Part model, mm, in its own coordinate system. Face numbers are marked on the shaded views. A direction names the side the tool comes from. Round coordinates to 2 decimals unless told otherwise and drop trailing zeros. Write each loop counter-clockwise with the first axis right and the second up, starting at its lowest first coordinate (ties: lowest second). Pieces come first, ordered by that corner, then holes. Notation, with made-up numbers: (-27, 77.25) -> (4, 77.25) arc R36 ccw to (4, 116.25) -> close; hole circle Ø7 at (-31.5, 12). An arc over 180 degrees is marked (long way). Return JSON: item names as keys, results as strings. Group by question number.
(1) Tool access for the marked faces 5, 6 and 7: list every direction of +Z, -Z, +X, -X, +Y, -Y with a clear straight run to the whole face (end or side of a thin tool).
(2) Saw through at A-A (y = 0). List the corners of the cut face in (x, z) (3 decimals), plus the area to 3 significant figures.
(3) Saw through at C-C (z = 1.9). State how many separate pieces and enclosed holes the cut face has, plus the area to 3 significant figures.
(4) Drill centre lines: L1, parallel to Y at x = 14.85, z = 2.25 (3 decimals); L2, parallel to X at y = 7.25, z = 1.5 (3 decimals); L3, parallel to Y at x = -6, z = 0.3 (3 decimals). Where is each one in solid material? Low to high. Write a range as from..to.
(5) Mould opens along Y. For the marked faces 1, 2, 3 and 4 say: +Y half, -Y half, draft (parallel to the pull), parting line (faces both ways), or undercut.
(6) Saw through at B-B (x = 0). List the corners of the cut face in (y, z) (3 decimals).
(7) Drop flat-ended pins along their axis: pin 1 Ø2.5 at (x, y) = (-14.375, 11.375) entering from -Z; pin 2 Ø2.5 at (y, z) = (5.49, 2.25) entering from +X (3 decimals); pin 3 Ø1 at (x, y) = (0.5, -6.5) entering from +Z; pin 4 Ø1.6 at (x, z) = (0, 4) entering from -Y. Give the stop position or say it passes through.
Autodesk Inventor part; units mm, degrees
ref_plane "YZ Plane" through (0, 0, 0) normal (1, 0, 0) x (0, 1, 0)
ref_plane "XZ Plane" through (0, 0, 0) normal (0, 1, 0) x (-1, 0, 0)
ref_plane "XY Plane" through (0, 0, 0) normal (0, 0, 1) x (1, 0, 0)
ref_plane "Work Plane1" through (0, 0, 0) normal (0, 0, 1) x (1, 0, 0)
sketch "Sketch1" plane through (0, 0, 0) normal (0, 0, 1) x (1, 0, 0)
  arc A0 (5.9062, 3.651) -> (7.7035, 4.7619) centre (6.8048, 4.2064) ccw
  arc A1 (5.9062, 3.651) -> (2.5768, 6.4477) centre (0, 0) ccw
  arc A2 (3.3608, 8.4097) -> (2.5768, 6.4477) centre (2.9688, 7.4287) ccw
  arc A3 (7.7035, 4.7619) -> (3.3608, 8.4097) centre (0, 0) ccw
  arc A4 (2.5768, -6.4477) -> (3.3608, -8.4097) centre (2.9688, -7.4287) ccw
  arc A5 (2.5768, -6.4477) -> (5.9062, -3.651) centre (0, 0) ccw
  arc A6 (7.7035, -4.7619) -> (5.9062, -3.651) centre (6.8048, -4.2064) ccw
  arc A7 (3.3608, -8.4097) -> (7.7035, -4.7619) centre (0, 0) ccw
  arc A8 (-2.5553, 6.4563) -> (-3.3328, 8.4209) centre (-2.9441, 7.4386) ccw
  arc A9 (-2.5553, 6.4563) -> (-5.9062, 3.651) centre (0, 0) ccw
  arc A10 (-7.7035, 4.7619) -> (-5.9062, 3.651) centre (-6.8048, 4.2064) ccw
  arc A11 (-3.3328, 8.4209) -> (-7.7035, 4.7619) centre (0, 0) ccw
  arc A12 (-5.9062, -3.651) -> (-7.7035, -4.7619) centre (-6.8048, -4.2064) ccw
  arc A13 (-5.9062, -3.651) -> (-2.5553, -6.4563) centre (0, 0) ccw
  arc A14 (-3.3328, -8.4209) -> (-2.5553, -6.4563) centre (-2.9441, -7.4386) ccw
  arc A15 (-7.7035, -4.7619) -> (-3.3328, -8.4209) centre (0, 0) ccw
  circle A16 centre (0.0124, -10.65) radius 1.15
  circle A17 centre (8, 0) radius 1.0564
  circle A18 centre (-8, 0) radius 1.0564
  circle A19 centre (0, 0) radius 5
  circle A20 centre (0, 0) radius 13.7
  line L0 (16.125, 14.375) -> (-17.375, 14.375)
  line L1 (-17.375, 14.375) -> (-17.375, -14.375)
  line L2 (-17.375, -14.375) -> (16.125, -14.375)
  line L3 (16.125, -14.375) -> (16.125, 14.375)
  circle A21 centre (0, 0) radius 13.7
  circle A22 centre (0, 0) radius 5.15
  arc A23 (5.4809, 3.3881) -> (8.1288, 5.0248) centre (6.8048, 4.2064) ccw
  arc A24 (5.4809, 3.3881) -> (2.3912, 5.9835) centre (0, 0) ccw
  arc A25 (3.5464, 8.874) -> (2.3912, 5.9835) centre (2.9688, 7.4287) ccw
  arc A26 (8.1288, 5.0248) -> (3.5464, 8.874) centre (0, 0) ccw
  arc A27 (8.1288, -5.0248) -> (5.4809, -3.3881) centre (6.8048, -4.2064) ccw
  arc A28 (2.3912, -5.9835) -> (5.4809, -3.3881) centre (0, 0) ccw
  arc A29 (2.3912, -5.9835) -> (3.5464, -8.874) centre (2.9688, -7.4287) ccw
  arc A30 (3.5464, -8.874) -> (8.1288, -5.0248) centre (0, 0) ccw
  circle A31 centre (0.0124, -10.65) radius 1.65
  arc A32 (-5.4809, -3.3881) -> (-2.3713, -5.9914) centre (0, 0) ccw
  arc A33 (-5.4809, -3.3881) -> (-8.1288, -5.0248) centre (-6.8048, -4.2064) ccw
  arc A34 (-8.1288, -5.0248) -> (-3.5168, -8.8858) centre (0, 0) ccw
  arc A35 (-3.5168, -8.8858) -> (-2.3713, -5.9914) centre (-2.9441, -7.4386) ccw
  arc A36 (-2.3713, 5.9914) -> (-5.4809, 3.3881) centre (0, 0) ccw
  arc A37 (-2.3713, 5.9914) -> (-3.5168, 8.8858) centre (-2.9441, 7.4386) ccw
  arc A38 (-3.5168, 8.8858) -> (-8.1288, 5.0248) centre (0, 0) ccw
  arc A39 (-8.1288, 5.0248) -> (-5.4809, 3.3881) centre (-6.8048, 4.2064) ccw
  circle A40 centre (-14.375, -11.375) radius 1.75
  circle A41 centre (13.125, 11.375) radius 1.75
  circle A42 centre (13.125, -11.375) radius 1.75
  circle A43 centre (-14.375, 11.375) radius 1.75
  point P0 (0, 0)
  dimension "d0" = 0.15
  dimension "d1" = 0.5
  dimension "d2" = 0.5
  dimension "d3" = 0.5
  dimension "d4" = 0.5
  dimension "d5" = 0.5
extrude "Extrusion1" add sketch "Sketch1" along normal blind 1.5 contours A20 | L3 L2 L1 L0 | A40 | A41 | A42 | A43
sketch "Sketch2" plane through (0, 0, 1.5) normal (0, 0, 1) x (1, 0, 0)
  line L0 (-17.375, 14.375) -> (-17.375, -14.375)
  line L1 (-17.375, -14.375) -> (16.125, -14.375)
  line L2 (16.125, -14.375) -> (16.125, 14.375)
  line L3 (16.125, 14.375) -> (-17.375, 14.375)
  circle A0 centre (8, 0) radius 1.0564
  circle A1 centre (-8, 0) radius 1.0564
  circle A2 centre (0, 0) radius 5.15
  arc A3 (5.4809, 3.3881) -> (2.3912, 5.9835) centre (0, 0) ccw
  arc A4 (3.5464, 8.874) -> (2.3912, 5.9835) centre (2.9688, 7.4287) ccw
  arc A5 (8.1288, 5.0248) -> (3.5464, 8.874) centre (0, 0) ccw
  arc A6 (5.4809, 3.3881) -> (8.1288, 5.0248) centre (6.8048, 4.2064) ccw
  arc A7 (2.3912, -5.9835) -> (5.4809, -3.3881) centre (0, 0) ccw
  arc A8 (8.1288, -5.0248) -> (5.4809, -3.3881) centre (6.8048, -4.2064) ccw
  arc A9 (3.5464, -8.874) -> (8.1288, -5.0248) centre (0, 0) ccw
  arc A10 (2.3912, -5.9835) -> (3.5464, -8.874) centre (2.9688, -7.4287) ccw
  circle A11 centre (0.0124, -10.65) radius 1.65
  arc A12 (-5.4809, -3.3881) -> (-8.1288, -5.0248) centre (-6.8048, -4.2064) ccw
  arc A13 (-5.4809, -3.3881) -> (-2.3713, -5.9914) centre (0, 0) ccw
  arc A14 (-3.5168, -8.8858) -> (-2.3713, -5.9914) centre (-2.9441, -7.4386) ccw
  arc A15 (-8.1288, -5.0248) -> (-3.5168, -8.8858) centre (0, 0) ccw
  arc A16 (-2.3713, 5.9914) -> (-3.5168, 8.8858) centre (-2.9441, 7.4386) ccw
  arc A17 (-2.3713, 5.9914) -> (-5.4809, 3.3881) centre (0, 0) ccw
  arc A18 (-8.1288, 5.0248) -> (-5.4809, 3.3881) centre (-6.8048, 4.2064) ccw
  arc A19 (-3.5168, 8.8858) -> (-8.1288, 5.0248) centre (0, 0) ccw
  arc A20 (8.1288, -5.0248) -> (5.4809, -3.3881) centre (6.8048, -4.2064) ccw
  line L4 (8.3613, -4.2064) -> (8.3613, -14.375)
  line L5 (-17.375, -14.375) -> (16.125, -14.375)
  arc A21 (-5.4809, -3.3881) -> (-8.1288, -5.0248) centre (-6.8048, -4.2064) ccw
  line L6 (-8.3613, -4.2064) -> (-8.3613, -14.375)
  arc A22 (2.3912, -5.9835) -> (3.5464, -8.874) centre (2.9688, -7.4287) ccw
  line L7 (1.6624, -6.5827) -> (-1.6441, -6.5827)
  arc A23 (-3.5168, -8.8858) -> (-2.3713, -5.9914) centre (-2.9441, -7.4386) ccw
  point P0 (0, 0)
extrude "Extrusion2" add sketch "Sketch2" along normal blind 1.5 contours L3 L2 L1 L4 A8 A7 A10 L7 A14 A13 A12 L6 L0
sketch "Sketch3" plane through (0, 0, 3) normal (0, 0, 1) x (1, 0, 0)
  circle A0 centre (0, 0) radius 6.75
  line L0 (-17.375, -14.375) -> (-8.3613, -14.375)
  line L1 (-8.3613, -14.375) -> (-8.3613, -4.2064)
  arc A1 (-5.4809, -3.3881) -> (-8.3613, -4.2064) centre (-6.8048, -4.2064) ccw
  arc A2 (-5.4809, -3.3881) -> (-2.3713, -5.9914) centre (0, 0) ccw
  arc A3 (-1.6441, -6.5827) -> (-2.3713, -5.9914) centre (-2.9441, -7.4386) ccw
  line L2 (-1.6441, -6.5827) -> (1.6624, -6.5827)
  arc A4 (2.3912, -5.9835) -> (1.6624, -6.5827) centre (2.9688, -7.4287) ccw
  arc A5 (2.3912, -5.9835) -> (5.4809, -3.3881) centre (0, 0) ccw
  arc A6 (8.3613, -4.2064) -> (5.4809, -3.3881) centre (6.8048, -4.2064) ccw
  line L3 (8.3613, -4.2064) -> (8.3613, -14.375)
  line L4 (8.3613, -14.375) -> (16.125, -14.375)
  line L5 (16.125, -14.375) -> (16.125, 14.375)
  line L6 (16.125, 14.375) -> (-17.375, 14.375)
  line L7 (-17.375, 14.375) -> (-17.375, -14.375)
  circle A7 centre (8, 0) radius 1.0564
  circle A8 centre (-8, 0) radius 1.0564
  arc A9 (-2.3713, 5.9914) -> (-5.4809, 3.3881) centre (0, 0) ccw
  arc A10 (-8.1288, 5.0248) -> (-5.4809, 3.3881) centre (-6.8048, 4.2064) ccw
  arc A11 (-3.5168, 8.8858) -> (-8.1288, 5.0248) centre (0, 0) ccw
  arc A12 (-2.3713, 5.9914) -> (-3.5168, 8.8858) centre (-2.9441, 7.4386) ccw
  arc A13 (5.4809, 3.3881) -> (8.1288, 5.0248) centre (6.8048, 4.2064) ccw
  arc A14 (5.4809, 3.3881) -> (2.3912, 5.9835) centre (0, 0) ccw
  arc A15 (3.5464, 8.874) -> (2.3912, 5.9835) centre (2.9688, 7.4287) ccw
  arc A16 (8.1288, 5.0248) -> (3.5464, 8.874) centre (0, 0) ccw
  circle A17 centre (0, 0) radius 5.15
  circle A18 centre (8, 0) radius 2.5
  circle A19 centre (-8, 0) radius 2.5
  line L8 (2.9688, 8.9852) -> (-2.9441, 8.9852)
  line L9 (2.9688, 8.9852) -> (8.8817, 8.9852) construction
  arc A20 (-8.1288, 5.0248) -> (-5.4809, 3.3881) centre (-6.8048, 4.2064) ccw
  line L10 (-8.3613, 4.2064) -> (-8.3613, -4.2064)
  arc A21 (-5.4809, -3.3881) -> (-8.1288, -5.0248) centre (-6.8048, -4.2064) ccw
  arc A22 (5.4809, 3.3881) -> (8.1288, 5.0248) centre (6.8048, 4.2064) ccw
  line L11 (8.3613, 4.2064) -> (8.3613, -4.2064)
  point P0 (0, 0)
  point P1 (-8.3613, -2.4738)
  point P2 (-8.3613, 2.4738)
  point P3 (-2.7693, 8.9852)
  point P4 (8.3613, 2.4738)
  point P5 (8.3613, -2.4738)
  dimension "d10" = 5
  dimension "d11" = 5
  dimension "d12" = 180
extrude "Extrusion3" add sketch "Sketch3" along normal blind 1.5 contours L11 A13 A16 A15 L8 A12 A11 A10 L10 A19 L1 L0 L7 L6 L5 L4 L3 A18
sketch "Sketch4" plane through (0, 0, 4.5) normal (0, 0, 1) x (1, 0, 0)
  line L0 (16.125, -14.375) -> (16.125, 14.375)
  line L1 (-17.375, -14.375) -> (16.125, -14.375)
  line L2 (16.125, 14.375) -> (12.625, 14.375)
  line L3 (12.625, -14.375) -> (16.125, -14.375)
  line L4 (16.125, -14.375) -> (16.125, 14.375)
  circle A0 centre (13.125, 11.375) radius 3
  circle A1 centre (13.125, -11.375) radius 3
  circle A2 centre (-14.375, -11.375) radius 3
  circle A3 centre (-14.375, 11.375) radius 3
  line L5 (-8.3613, -14.375) -> (-8.3613, -2.4738)
  arc A4 (-8.3613, 2.4738) -> (-8.3613, -2.4738) centre (-8, 0) ccw
  line L6 (-8.3613, 2.4738) -> (-8.3613, 4.2064)
  arc A5 (-8.1288, 5.0248) -> (-8.3613, 4.2064) centre (-6.8048, 4.2064) ccw
  arc A6 (-3.5168, 8.8858) -> (-8.1288, 5.0248) centre (0, 0) ccw
  arc A7 (-2.7693, 8.9852) -> (-3.5168, 8.8858) centre (-2.9441, 7.4386) ccw
  line L7 (-2.7693, 8.9852) -> (2.9688, 8.9852)
  arc A8 (3.5464, 8.874) -> (2.9688, 8.9852) centre (2.9688, 7.4287) ccw
  arc A9 (8.1288, 5.0248) -> (3.5464, 8.874) centre (0, 0) ccw
  arc A10 (8.3613, 4.2064) -> (8.1288, 5.0248) centre (6.8048, 4.2064) ccw
  line L8 (8.3613, 4.2064) -> (8.3613, 2.4738)
  arc A11 (8.3613, -2.4738) -> (8.3613, 2.4738) centre (8, 0) ccw
  line L9 (8.3613, -2.4738) -> (8.3613, -14.375)
  line L10 (8.3613, -14.375) -> (16.125, -14.375)
  line L11 (16.125, -14.375) -> (16.125, 14.375)
  line L12 (16.125, 14.375) -> (-17.375, 14.375)
  line L13 (-17.375, 14.375) -> (-17.375, -14.375)
  line L14 (-17.375, -14.375) -> (-8.3613, -14.375)
  point P0 (0, 0)
  dimension "d16" = 6
  dimension "d17" = 6
  dimension "d18" = 6
  dimension "d19" = 6
hole "Hole1" at (13.125, 11.375, 4.5) at (13.125, -11.375, 4.5) at (-14.375, -11.375, 4.5) at (-14.375, 11.375, 4.5) direction (0, 0, -1) diameter 2.9 end through all countersink diameter 5 countersink angle 90
sketch "Sketch5" plane through (16.125, -14.375, 0) normal (1, 0, 0) x (0, 0, -1)
  line L0 (0, 27.2) -> (0, 24.3)
  line L1 (-3.45, 27.2) -> (-3.45, 24.3)
  line L2 (0, 4.45) -> (0, 1.55)
  line L3 (-3.45, 4.45) -> (-3.45, 1.55)
  line L4 (0, 0) -> (0, 28.75)
  line L5 (-4.5, 0) -> (-4.5, 28.75)
  line L6 (0, 28.75) -> (-4.5, 28.75)
  line L7 (-4.5, 28.75) -> (-4.5, 24.3)
  line L8 (-4.5, 24.3) -> (0, 24.3)
  line L9 (0, 24.3) -> (0, 28.75)
  line L10 (0, 0) -> (-4.5, 0)
  line L11 (-4.5, 0) -> (-4.5, 4.45)
  line L12 (-4.5, 4.45) -> (0, 4.45)
  line L13 (0, 4.45) -> (0, 0)
  line L14 (2.8, 13.3186) -> (0, 13.3186)
  line L15 (2.8, 15.4314) -> (0, 15.4314)
  line L16 (0, 15.4314) -> (-4.5, 15.4314)
  line L17 (-4.5, 15.4314) -> (-4.5, 13.3186)
  line L18 (-4.5, 13.3186) -> (0, 13.3186)
  line L19 (0, 13.3186) -> (0, 15.4314)
  line L20 (0, 24.3) -> (-4.5, 15.4314)
  line L21 (-4.5, 13.3186) -> (0, 4.45)
  line L22 (-4.5, 4.45) -> (0, 13.3186)
  line L23 (0, 13.3186) -> (0, 15.4314)
  line L24 (-4.5, 24.3) -> (0, 15.4314)
  point P0 (0, 14.375)
  point P1 (-2.25, 19.8657)
  point P2 (-2.25, 8.8843)
hole "Hole2" at (16.125, 5.4907, 2.25) at (16.125, -5.4907, 2.25) direction (-1, 0, 0) diameter 3 depth 3 counterbore diameter 3.5 counterbore depth 0.4
properties part number "right_motor_front_mount" material "Nylon 6/6"
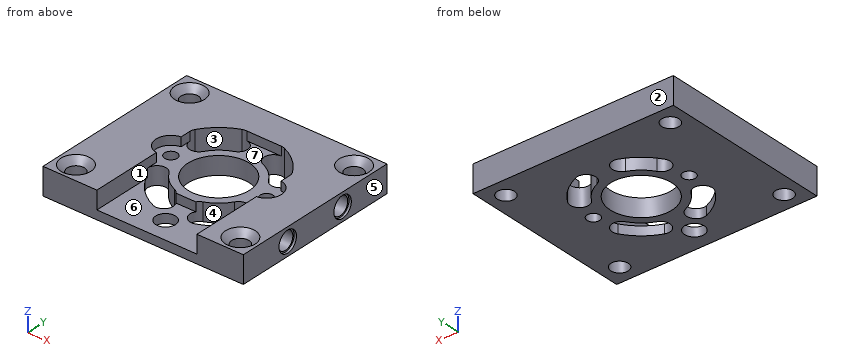
Computed values:
{
 "1": {"face 5": "+Z, -Z, +X, +Y, -Y", "face 6": "+Z, -Y", "face 7": "+Z"},
 "2": {"outline": "(-17.375, 0) -> (-9.056, 0) -> (-9.056, 3) -> (-10.5, 3) -> (-10.5, 4.5) -> (-17.375, 4.5) -> close; (-6.944, 0) -> (-5.15, 0) -> (-5.15, 3) -> (-6.944, 3) -> close; (5.15, 0) -> (6.944, 0) -> (6.944, 3) -> (5.15, 3) -> close; (9.056, 0) -> (16.125, 0) -> (16.125, 4.5) -> (10.5, 4.5) -> (10.5, 3) -> (9.056, 3) -> close", "area": "75.7 mm2"},
 "3": {"separate pieces": "1", "enclosed holes": "9", "area": "620 mm2"},
 "4": {"L1": "-14.375..-6.991, -3.991..3.991, 6.991..14.375", "L2": "-17.375..-6.226, -1.399..1.423, 6.226..16.125", "L3": "-14.375..-7.438, -2.874..2.874, 7.438..14.375"},
 "5": {"face 1": "draft", "face 2": "+Y half", "face 3": "undercut", "face 4": "undercut"},
 "6": {"outline": "(-14.375, 0) -> (-12.3, 0) -> (-12.3, 1.5) -> (-14.375, 1.5) -> close; (-9, 0) -> (-5.15, 0) -> (-5.15, 3) -> (-6.583, 3) -> (-6.583, 1.5) -> (-9, 1.5) -> close; (5.15, 0) -> (14.375, 0) -> (14.375, 4.5) -> (8.985, 4.5) -> (8.985, 3) -> (5.15, 3) -> close"},
 "7": {"pin 1": "through", "pin 2": "x = 13.125", "pin 3": "z = 3", "pin 4": "y = 8.99"}
}
